from build123d import *

# Parameters (mm, degrees)
SKETCH1_W               = 20
SKETCH1_H               = 20
BOSS_EXTRUDE1_DEPTH     = 4
CUT_EXTRUDE1_DEPTH      = 3
SKETCH1_4_R             = 2.1
CUT_EXTRUDE2_DEPTH      = 5
CUT_EXTRUDE2_DEPTH_BACK = 1


with BuildPart() as part:
    # Sketch1 → Boss-Extrude1 (new body)
    with BuildSketch(Plane(origin=(0, 0, 0), x_dir=(1, 0, 0), z_dir=(0, 1, 0))):
        Rectangle(SKETCH1_W, SKETCH1_H)
    extrude(amount=BOSS_EXTRUDE1_DEPTH)

    # Sketch1<3> → Cut-Extrude1 (cut)
    with BuildSketch(Plane(origin=(0, 0, 0), x_dir=(1, 0, 0), z_dir=(0, 1, 0))):
        Polygon((0, 4.041451884), (-3.5, 2.020725942), (-3.5, -2.020725942), (0, -4.041451884), (3.5, -2.020725942), (3.5, 2.020725942), align=None)
    extrude(amount=CUT_EXTRUDE1_DEPTH, mode=Mode.SUBTRACT)

    # Sketch1<4> → Cut-Extrude2 (cut, two sides)
    with BuildSketch(Plane(origin=(0, 0, 0), x_dir=(1, 0, 0), z_dir=(0, 1, 0))) as cut_extrude2_sk:
        Circle(SKETCH1_4_R)
    extrude(amount=CUT_EXTRUDE2_DEPTH, mode=Mode.SUBTRACT)
    extrude(cut_extrude2_sk.sketch, amount=-CUT_EXTRUDE2_DEPTH_BACK, mode=Mode.SUBTRACT)


solid = part.part
For this review, take the finished solid that the model builds, in its own axes (mm). A direction names the side the tool comes from. Coordinates: 2 decimals unless noted, no trailing zeros. Write each loop counter-clockwise with the first axis right and the second up, starting at its lowest first coordinate (ties: lowest second). Pieces come first, ordered by that corner, then holes. Notation, with made-up numbers: (27.5, -6.5) -> (34.5, -6.5) arc R18 ccw to (34.5, 8.5) -> close; hole circle Ø6 at (14, 56). An arc over 180 degrees is marked (long way). Write each question's results on one line, items separated by ' | '. Start each with the question number.
1) Insertion check: pin 1 (2.5 mm diameter, centred on x = 0, z = 0, fed in from -Y). The pin has a flat end and moves straight along its axis. Give the tip position at first contact, or say it passes through.
2) Wall thickness on L1, parallel to Z at x = 0, y = 3.3; L2, parallel to X at y = 2.65, z = 0.25; L3, parallel to Y at x = -0.75, z = -2.5: over which ranges is each line inside the solid? List them lowest first. Write a range as [from, to].
3) The part is to be moulded in two halves that separate along X. For faces 1 (the face through (-10, 2, 0)), 2 (the face through (-3.5, 1, 0)), 3 (the face through (4, 0, 0)), 4 (the face through (1.8, 1.5, -3)), say which applies: +X half, -X half, draft (parallel to the pull), parting line (faces both ways), or undercut.
4) For faces 5 (the face through (-2, 3, 2)), 6 (the face through (2.003, 3.493, -0.631)), list the 3-axis set-ups (+Z, -Z, +X, -X, +Y, -Y) from which the entire face can be reached by the end or side of a thin tool; tool diameter is ignored.
5) Consider section A-A (z = 0). Write out the cut boundary in (x, y).
6) Consider section D-D (y = 0.95). Write out the cut boundary in (x, z), plus the area to 3 significant figures.
7) Consider section B-B (y = 3.5). Write out the cut boundary in (x, z), plus the area to 3 significant figures.
8) Consider section C-C (x = -3). Write out the cut boundary in (y, z), plus the area to 3 significant figures.
Geometry says:
1) pin 1: through
2) L1: [-10, -2.1], [2.1, 10] | L2: [-10, -3.5], [3.5, 10] | L3: [3, 4]
3) face 1: -X half | face 2: undercut | face 3: draft | face 4: undercut
4) face 5: -Y | face 6: +Y, -Y
5) outline: (-10, 0) -> (-3.5, 0) -> (-3.5, 3) -> (-2.1, 3) -> (-2.1, 4) -> (-10, 4) -> close; (2.1, 3) -> (3.5, 3) -> (3.5, 0) -> (10, 0) -> (10, 4) -> (2.1, 4) -> close
6) outline: (-10, -10) -> (10, -10) -> (10, 10) -> (-10, 10) -> close; hole (-3.5, -2.02) -> (0, -4.04) -> (3.5, -2.02) -> (3.5, 2.02) -> (0, 4.04) -> (-3.5, 2.02) -> close | area: 358 mm^2
7) outline: (-10, -10) -> (10, -10) -> (10, 10) -> (-10, 10) -> close; hole circle Ø4.2 at (0, 0) | area: 386 mm^2
8) outline: (0, -10) -> (4, -10) -> (4, 10) -> (0, 10) -> (0, 2.31) -> (3, 2.31) -> (3, -2.31) -> (0, -2.31) -> close | area: 66.1 mm^2
